from build123d import *

# Parameters (mm, degrees)
EXTRUDE_1_DEPTH              = 7
CUT_EXTRUDE_1_DEPTH          = 4
HOLE_WIZARD_M3_1_D           = 3.4
HOLE_WIZARD_M3_1_DEPTH       = 7.5
HOLE_WIZARD_M3_1_CSINK_D     = 6.72
HOLE_WIZARD_M3_1_CSINK_ANGLE = 90
HOLE_WIZARD_M3_1_TIP         = 1.021463052
HOLE_WIZARD_1_D              = 4.15
CUT_EXTRUDE_2_DEPTH          = 4


with BuildPart() as part:
    # 草图1 → 凸台-拉伸1 (new body)
    with BuildSketch(Plane(origin=(0, 0, 0), x_dir=(1, 0, 0), z_dir=(0, 1, 0))):
        with BuildLine():
            Line((-4.5, 5), (4.5, 5))
            ThreePointArc((4.5, 5), (9.5, 0), (4.5, -5))
            Line((4.5, -5), (-4.5, -5))
            ThreePointArc((-4.5, -5), (-9.5, 0), (-4.5, 5))
        make_face()
    extrude(amount=EXTRUDE_1_DEPTH)

    # 草图2 → 切除-拉伸1 (cut)
    with BuildSketch(Plane(origin=(0, 7, 0), x_dir=(1, 0, 0), z_dir=(0, 1, 0))):
        with BuildLine():
            Line((-3, 2), (-6, 2))
            ThreePointArc((-6, 2), (-7, 0), (-6, -2))
            Line((-6, -2), (-3, -2))
            ThreePointArc((-3, -2), (-2.263932023, -1.118033989), (-2, 0))
            ThreePointArc((-2, 0), (-2.263932023, 1.118033989), (-3, 2))
        make_face()
    extrude(amount=-CUT_EXTRUDE_1_DEPTH, mode=Mode.SUBTRACT)

    # M3 六角凹锥坑螺钉的锥形沉头孔1
    with Locations(Plane(origin=(0, 0, 0), x_dir=(-1, 0, 0), z_dir=(0, -1, 0))):
        with Locations((4.5, 0)):
            CounterSinkHole(HOLE_WIZARD_M3_1_D / 2, HOLE_WIZARD_M3_1_CSINK_D / 2, depth=HOLE_WIZARD_M3_1_DEPTH, counter_sink_angle=HOLE_WIZARD_M3_1_CSINK_ANGLE)
            with Locations((0, 0, -(HOLE_WIZARD_M3_1_DEPTH + HOLE_WIZARD_M3_1_TIP / 2))):  # 118° drill point
                Cone(0, HOLE_WIZARD_M3_1_D / 2, HOLE_WIZARD_M3_1_TIP, mode=Mode.SUBTRACT)

    # 孔1 (through all)
    with Locations(Plane(origin=(0, 7, 0), x_dir=(1, 0, 0), z_dir=(0, 1, 0))):
        with Locations((5, -0.436816998)):
            Hole(HOLE_WIZARD_1_D / 2)

    # 草图12 → 切除-拉伸2 (cut)
    with BuildSketch(Plane(origin=(0, 7, 0), x_dir=(1, 0, 0), z_dir=(0, 1, 0))):
        Polygon((8.348631561, -0.436816998), (6.674315781, 2.463183002), (3.325684219, 2.463183002), (1.651368439, -0.436816998), (3.325684219, -3.336816998), (6.674315781, -3.336816998), align=None)
    extrude(amount=-CUT_EXTRUDE_2_DEPTH, mode=Mode.SUBTRACT)


solid = part.part
Check sheet for the modelled part. Datum: model origin and axes. Units: mm. A direction names the side the tool comes from. Round coordinates to 2 decimals unless told otherwise and drop trailing zeros. Order: outer loops, then holes, each group sorted by start corner. A loop starts at its lowest first (then second) coordinate and runs counter-clockwise, first axis right, second up.
(1) Scan lines: probe 1 along Z at (x, y) = (-4.5, 2.2); probe 2 along X at (y, z) = (4.25, -1.75); probe 3 along Y at (x, z) = (3.25, -0.75). Record each from-to range of solid material in increasing order.
(2) Access from +Z, -Z, +X, -X, +Y, -Y to the whole of each face (thin tool, end or side, straight path). Record for faces 4 (the cylindrical face through (-2.93, 2.34, 0.65)), 5 (the cylindrical face through (-7, 5, 0)).
(3) Cross-section at A-A, the plane x = 5. Enter the section's corners in (y, z).
(4) Cross-section at B-B, the plane x = 7.75. Enter the section's corners in (y, z).
(5) Go/stop test with flat-tipped pins: P1, Ø1, axis at x = -7.5, y = 4.5, coming from the +Z side; P2, Ø1.5, axis at y = 5, z = -2, coming from the -X side. Record where each tip stops, or that it passes through.
(6) Cross-section at C-C, the plane z = -0.5. State how many separate pieces and enclosed holes the cut face has, and give its area (3 significant figures).
(7) Cross-section at D-D, the plane z = -4. Enter the section's corners in (x, y), and give its area (3 significant figures).
(8) Draft check along Z on faces 1 (the flat face through (5, 5, -2.463)), 2 (the cylindrical face through (-9.5, 3.5, 0.1)), 3 (the flat face through (0, 3, 5)). Enter one of: pulls with the +Z half, pulls with the -Z half, needs draft (parallel to the pull), parting line crosses it, or undercut.
Check sheet entries:
1. probe 1: z = -5 to -1.7, 1.7 to 5
1. probe 2: x = -9.18 to -6.29, -2.71 to 2.91, 7.09 to 9.18
1. probe 3: y = 0 to 3
2. face 4: +Y, -Y
2. face 5: +Y
3. outline: (0, -4.97) - (7, -4.97) - (7, -2.46) - (3, -2.46) - (3, -1.64) - (0, -1.64) - close; (0, 2.51) - (3, 2.51) - (3, 3.34) - (7, 3.34) - (7, 4.97) - (0, 4.97) - close
4. outline: (0, -3.8) - (7, -3.8) - (7, -0.6) - (3, -0.6) - (3, 1.47) - (7, 1.47) - (7, 3.8) - (0, 3.8) - close
5. P1: stops at z = 4.33
5. P2: stops at x = -9.34
6. separate pieces: 3
6. enclosed holes: 0
6. area: 66.9 mm2
7. outline: (-7.5, 0) - (7.5, 0) - (7.5, 7) - (-7.5, 7) - close
7. area: 105 mm2
8. face 1: undercut
8. face 2: parting line crosses it
8. face 3: pulls with the +Z half
